from build123d import *

# Parameters (mm, degrees)
F0_W     = 40
F0_H     = 6
F1_DEPTH = 90
F4_D     = 9
F5_W     = 6
F5_H     = 36.9851887226
F5_H_2   = 204.6339064837
F5_H_3   = 206.7867070436
F5_H_4   = 36.1703634262
F6_DEPTH = 18
F7_DEPTH = 15


# Not quite as in the source:
# - a feature names something its author has since deleted; it is built from what else it names


with BuildPart() as f1:
    # F0 (on Right) → F1 (new body)
    with BuildSketch(Plane.YZ):
        with Locations((-0.72813743, 3)):
            Rectangle(F0_W, F0_H)
    extrude(amount=F1_DEPTH)

    # F4 (through all)
    with Locations(Plane(origin=(0, 0, 0), x_dir=(1, 0, 0), z_dir=(0, 0, -1))):
        with Locations((13, 0), (77, 0)):
            Hole(F4_D / 2)

    # F5 (on Front) → F6 (join)
    with BuildSketch(Plane.XZ):
        with Locations((62.4182647765, 235.9948903322)):
            Rectangle(F5_W, F5_H)
        Polygon((59.4182647765, 217.5022959709), (55.5, 204.6339064837), (61.5, 204.6339064837), (65.4182647765, 217.5022959709), align=None)
        with Locations((58.5, 102.3169532418)):
            Rectangle(F5_W, F5_H_2)
        with Locations((31.5, 103.3933535218)):
            Rectangle(F5_W, F5_H_3)
        Polygon((26.9661769271, 219.9091017246), (28.5, 206.7867070436), (34.5, 206.7867070436), (32.9661769271, 219.9091017246), align=None)
        with Locations((29.9661769271, 237.9942834377)):
            Rectangle(F5_W, F5_H_4)
    extrude(amount=F6_DEPTH)

    # F7 (add): faces of the model
    f7_faces = [f1.faces().sort_by_distance(p)[0] for p in [
        (31.2379126918, 0, 131.0397325754),
        (59.1846567788, 0, 130.2437423468),
    ]]
    extrude(f7_faces, amount=F7_DEPTH)


solid = f1.part
Geometry check sheet. Reference: the model listing, model coordinates, mm. A direction names the side the tool comes from. Coordinates: 2 decimals unless noted, no trailing zeros. Order: outer loops, then holes, each group sorted by start corner. A loop starts at its lowest first (then second) coordinate and runs counter-clockwise, first axis right, second up. Notation, with made-up numbers: (32.25, 85) - (50.25, 85) arc R21 ccw to (50.25, 105) - close; hole circle Ø6 at (67.25, 33.25). An arc over 180 degrees is marked (long way). Answer in a Markdown table with one row per item. Add a question column.
1) Set-up check for faces 1 (the flat face through (65.418, -1, 236)), 2 (the flat face through (57.5, -1.3, 211.2)), 3 (the flat face through (59, 15, 132)), 4 (the flat face through (27.722, -1.731, 213.44)): record each of +Z, -Z, +X, -X, +Y, -Y from which the full face is reachable in a straight line by a thin tool's end or side.
2) Release check for a two-part mould opening along Y. For faces 5 (the flat face through (32, -18, 133)), 6 (the cylindrical face through (8.708, -1.352, 3.042)), 7 (the flat face through (63.432, -1.269, 210.978)) record: +Y half, -Y half, draft (parallel to the pull), parting line (faces both ways), or undercut.
3) Material ranges on line 1 along X through (y, z) = (10.5, 156); line 2 along Y through (x, z) = (13, 2.25); line 3 along Z through (x, y) = (47, 2), recorded low to high. Write a range as [from, to].
4) Cross-section at B-B, the plane z = 196.5. Record the cut outline in (x, y), then the cut area to 3 significant figures.
5) Gauge pin test, flat ends, axial feed: P1, Ø10, axis at y = -7, z = 231, coming from the +X side; P2, Ø2, axis at x = 11, y = 8, coming from the +Z side; P3, Ø8, axis at x = 59.5, z = 177.5, coming from the +Y side. Record the tip position at first contact, or that the pin passes through.
6) Cross-section at D-D, the plane y = -11.5. Record the cut outline in (x, z).
7) Cross-section at A-A, the plane x = 13. Record the cut outline in (y, z).
8) Cross-section at C-C, the plane y = 0. Record the cut outline in (x, z).
Check result:
| question | item | result |
|---|---|---|
| 1 | face 1 | +Z, +X, +Y, -Y |
| 1 | face 2 | +Z, +Y, -Y |
| 1 | face 3 | +Z, +X, -X, +Y |
| 1 | face 4 | -X, +Y, -Y |
| 2 | face 5 | -Y half |
| 2 | face 6 | undercut |
| 2 | face 7 | draft |
| 3 | line 1 | x = [28.5, 34.5], [55.5, 61.5] |
| 3 | line 2 | y = [-20.73, -4.5], [4.5, 19.27] |
| 3 | line 3 | z = [0, 6] |
| 4 | outline | (28.5, -18) - (34.5, -18) - (34.5, 15) - (28.5, 15) - close; (55.5, -18) - (61.5, -18) - (61.5, 15) - (55.5, 15) - close |
| 4 | area | 396 mm² |
| 5 | P1 | stops at x = 65.42 |
| 5 | P2 | stops at z = 6 |
| 5 | P3 | stops at y = 15 |
| 6 | outline | (0, 0) - (90, 0) - (90, 6) - (61.5, 6) - (61.5, 204.63) - (65.42, 217.5) - (65.42, 254.49) - (59.42, 254.49) - (59.42, 217.5) - (55.5, 204.63) - (55.5, 6) - (34.5, 6) - (34.5, 206.79) - (32.97, 219.91) - (32.97, 256.08) - (26.97, 256.08) - (26.97, 219.91) - (28.5, 206.79) - (28.5, 6) - (0, 6) - close |
| 7 | outline | (-20.73, 0) - (-4.5, 0) - (-4.5, 6) - (-20.73, 6) - close; (4.5, 0) - (19.27, 0) - (19.27, 6) - (4.5, 6) - close |
| 8 | outline | (0, 0) - (8.5, 0) - (8.5, 6) - (0, 6) - close; (17.5, 0) - (72.5, 0) - (72.5, 6) - (61.5, 6) - (61.5, 204.63) - (65.42, 217.5) - (65.42, 254.49) - (59.42, 254.49) - (59.42, 217.5) - (55.5, 204.63) - (55.5, 6) - (34.5, 6) - (34.5, 206.79) - (32.97, 219.91) - (32.97, 256.08) - (26.97, 256.08) - (26.97, 219.91) - (28.5, 206.79) - (28.5, 6) - (17.5, 6) - close; (81.5, 0) - (90, 0) - (90, 6) - (81.5, 6) - close |
